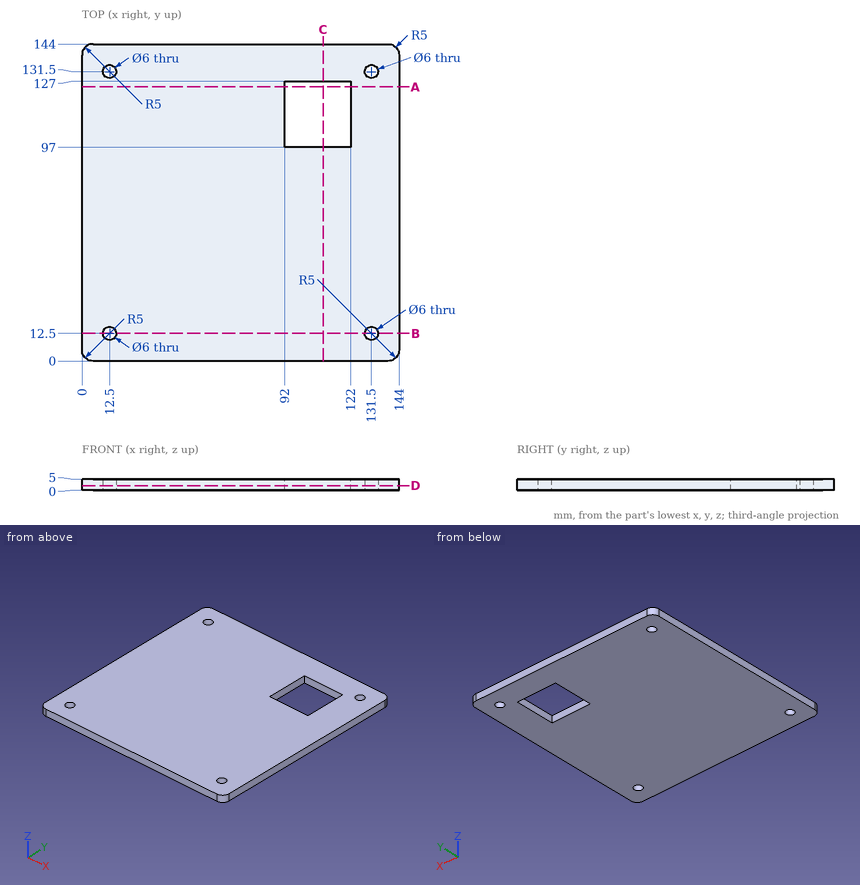
For this review, use the dimensioned drawing (mm, ordinates from the lowest corner) and the shaded views. Coordinates: 2 decimals unless noted, no trailing zeros. Loops run counter-clockwise (first coordinate to the right, second up) from the corner with the lowest first, then second, coordinate; pieces in that order, holes last. Notation, with made-up numbers: M 0.25,-7.5 L 9.25,-7.5 A25 ccw 9.25,13.5 Z; hole C -13.75,7.5 d10. An arc over 180 degrees is marked long. Answer as CSV lines item,"result".
Item 1: For probe 1 along X at (y, z) = (131.5, 3.05); probe 2 along X at (y, z) = (104.5, 0.75), list the stretches that pass through material, from the lowest coordinate up.
Answer list:
probe 1,"0 to 9.5, 15.5 to 128.5, 134.5 to 144"
probe 2,"0 to 92, 122 to 144"
Item 2: Add section B-B on y = 12.5. State the section outline as (x, z) points.
Answer list:
outline,"M 0,0 L 9.5,0 L 9.5,5 L 0,5 Z; M 15.5,0 L 128.5,0 L 128.5,5 L 15.5,5 Z; M 134.5,0 L 144,0 L 144,5 L 134.5,5 Z"
Item 3: Add section D-D on z = 1.95. State the section outline as (x, y) points, plus the area to 3 significant figures.
Answer list:
outline,"M 0,5 A5 ccw 5,0 L 139,0 A5 ccw 144,5 L 144,139 A5 ccw 139,144 L 5,144 A5 ccw 0,139 Z; hole C 12.5,12.5 d6; hole C 12.5,131.5 d6; hole M 92,97 L 122,97 L 122,127 L 92,127 Z; hole C 131.5,12.5 d6; hole C 131.5,131.5 d6"
area,"19,700 mm²"
Item 4: Add section C-C on x = 109.5. State the section outline as (y, z) points, plus the area to 3 significant figures.
Answer list:
outline,"M 0,0 L 97,0 L 97,5 L 0,5 Z; M 127,0 L 144,0 L 144,5 L 127,5 Z"
area,"570 mm²"
Item 5: For P1, Ø5, axis at x = 131.5, y = 131.5, coming from the -Z side, flat-tipped, find the tip position at first contact; note if it passes through.
Answer list:
P1,"through"
Item 6: Add section A-A on y = 124.5. State the section outline as (x, z) points, plus the area to 3 significant figures.
Answer list:
outline,"M 0,0 L 92,0 L 92,5 L 0,5 Z; M 122,0 L 144,0 L 144,5 L 122,5 Z"
area,"570 mm²"
